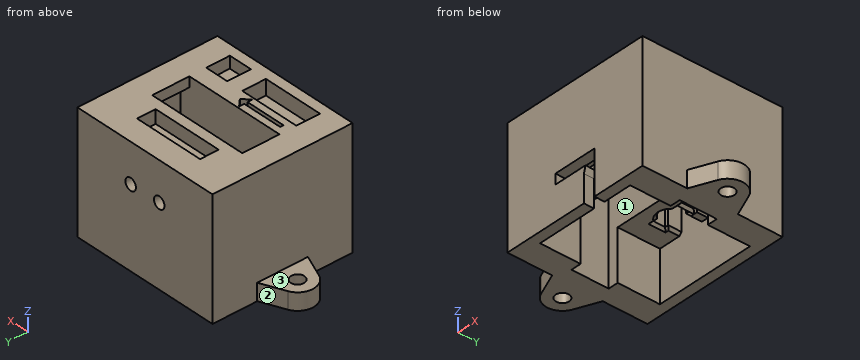
from build123d import *

# Parameters (mm, degrees)
F0_W      = 45
F0_H      = 41.5
F0_W_2    = 18
F0_H_2    = 4
F0_W_3    = 7
F0_H_3    = 3
F0_W_4    = 30
F0_H_4    = 11
F0_W_5    = 8
F0_H_5    = 3.5
F1_DEPTH  = 35
F2_W      = 21
F2_H      = 5.5
F3_DEPTH  = 4
F4_R      = 1.75
F5_DEPTH  = 25
F7_DEPTH  = 4
F9_START  = -8
F8_R      = 3.25
F9_DEPTH  = 17
F11_START = -3
F10_W     = 36
F10_H     = 11
F11_DEPTH = 32.001
F12_W     = 18
F12_H     = 7
F13_DEPTH = 4.5
F14_W     = 7
F14_H     = 4
F15_DEPTH = 3.5
F17_START = -20
F16_W     = 30
F16_H     = 12.5
F16_H_2   = 12
F17_DEPTH = 15.001
F19_DEPTH = 2
F20_R     = 2
F21_DEPTH = 5
F23_DEPTH = 10
F24_SIZE  = 0.74999


# Not quite as in the source:
# - a fillet or chamfer is up to 0.001 mm smaller than in the source, because OpenCascade refuses the exact size


with BuildPart() as f1:
    # F0 (on Top) → F1 (new body)
    with BuildSketch(Plane.XY):
        Rectangle(F0_W, F0_H)
        with Locations((-6, -12.75)):
            Rectangle(F0_W_2, F0_H_2, mode=Mode.SUBTRACT)
        with Locations((11.5, -12.25)):
            Rectangle(F0_W_3, F0_H_3, mode=Mode.SUBTRACT)
        with Locations((0, -0.25)):
            Rectangle(F0_W_4, F0_H_4, mode=Mode.SUBTRACT)
        with Locations((-4.75, 12)):
            Rectangle(F0_W_5, F0_H_5, mode=Mode.SUBTRACT)
        with Locations((4.75, 12)):
            Rectangle(F0_W_5, F0_H_5, mode=Mode.SUBTRACT)
    extrude(amount=F1_DEPTH)

    # F2 (on face) → F3 (cut)
    with BuildSketch(Plane.XY.offset(35)):
        with Locations((0, 11)):
            Rectangle(F2_W, F2_H)
    extrude(amount=-F3_DEPTH, mode=Mode.SUBTRACT)

    # F4 (on face) → F5 (cut)
    with BuildSketch(Plane.XZ.offset(-13.75)):
        with Locations((4.75, 23.5)):
            Circle(F4_R)
        with Locations((-4.75, 23.5)):
            Circle(F4_R)
    extrude(amount=-F5_DEPTH, mode=Mode.SUBTRACT)

    # F6 (on face) → F7 (cut)
    with BuildSketch(Plane.XZ.offset(-13.75)):
        Polygon((4.75, 26.9641016151), (1.75, 25.2320508076), (1.75, 21.7679491924), (1.75, -5.2918036282), (7.75, -5.2918036282), (7.75, 21.7679491924), (7.75, 25.2320508076), align=None)
        Polygon((-1.75, 21.7679491924), (-1.75, 25.2320508076), (-4.75, 26.9641016151), (-7.75, 25.2320508076), (-7.75, 21.7679491924), (-7.75, -5.2918036282), (-1.75, -5.2918036282), align=None)
    extrude(amount=-F7_DEPTH, mode=Mode.SUBTRACT)

    # F8 (on face) → F9 (cut)
    with BuildSketch(Plane.XY.offset(31).offset(F9_START)):
        with Locations((4.75, 12)):
            Circle(F8_R)
        with Locations((-4.75, 12)):
            Circle(F8_R)
    extrude(amount=-F9_DEPTH, mode=Mode.SUBTRACT)

    # F10 (on face) → F11 (cut)
    with BuildSketch(Plane.XY.offset(35).offset(F11_START)):
        with Locations((0, -0.25)):
            Rectangle(F10_W, F10_H)
    extrude(amount=-F11_DEPTH, mode=Mode.SUBTRACT)

    # F12 (on face) → F13 (cut)
    with BuildSketch(Plane.XY.offset(35)):
        with Locations((-6, -14.25)):
            Rectangle(F12_W, F12_H)
    extrude(amount=-F13_DEPTH, mode=Mode.SUBTRACT)

    # F14 (on face) → F15 (cut)
    with BuildSketch(Plane.XY.offset(35)):
        with Locations((11.5, -15.75)):
            Rectangle(F14_W, F14_H)
    extrude(amount=-F15_DEPTH, mode=Mode.SUBTRACT)

    # F16 (on face) → F17 (cut)
    with BuildSketch(Plane.XY.offset(35).offset(F17_START)):
        with Locations((0, 11.5)):
            Rectangle(F16_W, F16_H)
        with Locations((0, -11.75)):
            Rectangle(F16_W, F16_H_2)
    extrude(amount=-F17_DEPTH, mode=Mode.SUBTRACT)

    # F18 (on face) → F19 (cut)
    with BuildSketch(Plane.XY.offset(35)):
        Polygon((-1, -7.75), (-13, -7.75), (-13, -8.75), (-1, -8.75), (-1, -10.25), (1, -8.25), (-1, -6.25), align=None)
    extrude(amount=-F19_DEPTH, mode=Mode.SUBTRACT)

    # F20 (on Top) → F21 (join)
    with BuildSketch(Plane.XY):
        with BuildLine():
            Line((22.5, -7.5), (29.4230769231, -4.6153846154))
            ThreePointArc((29.4230769231, -4.6153846154), (32.5, 0), (29.4230769231, 4.6153846154))
            Line((29.4230769231, 4.6153846154), (22.5, 7.5))
            Line((22.5, 7.5), (22.5, -7.5))
        make_face()
        with Locations((27.5, 0)):
            Circle(F20_R, mode=Mode.SUBTRACT)
        with BuildLine():
            Line((-29.4230769231, -4.6153846154), (-22.5, -7.5))
            Line((-22.5, -7.5), (-22.5, 7.5))
            Line((-22.5, 7.5), (-29.4230769231, 4.6153846154))
            ThreePointArc((-29.4230769231, 4.6153846154), (-32.5, 0), (-29.4230769231, -4.6153846154))
        make_face()
        with Locations((-27.5, 0)):
            Circle(F20_R, mode=Mode.SUBTRACT)
    extrude(amount=F21_DEPTH)

    # F22 (on face) → F23 (cut)
    with BuildSketch(Plane.XZ.offset(20.75)):
        Polygon((3, 8), (3, 0), (6.5, 0), (6.5, 13), (-6.5, 13), (-6.5, 10), (3.5, 10), align=None)
    extrude(amount=-F23_DEPTH, mode=Mode.SUBTRACT)

    # F24 (size 0.75 in the source; OpenCascade refuses exactly that, so slightly less here)
    f24_edges = [f1.edges().sort_by_distance(p)[0] for p in [
        (-7.75, 15.75, 15),
        (-4.75, 8.75, 15),
        (8.119306, 10.25, 15),
        (1.380694, 10.25, 15),
        (-1.380694, 10.25, 15),
        (-8.119306, 10.25, 15),
        (-8.75, 12, 15),
        (-8.25, 13.75, 15),
        (-1.25, 13.75, 15),
        (1.25, 13.75, 15),
        (8.25, 13.75, 15),
        (-1.75, 15.75, 15),
        (1.75, 15.75, 15),
        (4.75, 8.75, 15),
        (8.75, 12, 15),
        (7.75, 15.75, 15),
        (-0.75, 12, 15),
        (0.75, 12, 15),
        (4.75, 10.25, 23),
        (-4.75, 10.25, 23),
    ]]
    chamfer(f24_edges, length=F24_SIZE)


solid = f1.part
Here's how the part is built. I have some questions about the finished solid (model axes, mm). Face numbers are marked on the shaded views. A direction names the side the tool comes from. Give positions to 0.01 mm unless a question says otherwise; leave off trailing zeros. Order: outer loops, then holes, each group sorted by start corner. A loop starts at its lowest first (then second) coordinate and runs counter-clockwise, first axis right, second up. Notation, with made-up numbers: (5.25, 62.5) -> (21.25, 62.5) arc R28 cw to (21.25, 96.5) -> close; hole circle Ø2 at (8, -24). An arc over 180 degrees is marked (long way). One line per item, written item: value. Start each with the question number.
1. Imagine slicing it at A-A, the plane y = 3. List the corners of the cut face in (x, z) for me, plus the area to 3 significant figures.
2. Will these pins go through, and if not, where does the flat tip stop? pin 1 Ø5 at (x, y) = (7.5, 10) entering from +Z; pin 2 Ø8 at (y, z) = (-2, 12) entering from +X; pin 3 Ø3 at (x, y) = (7.5, 8) entering from -Z; pin 4 Ø1.5 at (x, y) = (25.5, 5) entering from +Z.
3. Imagine slicing it at B-B, the plane z = 4. Count the separate pieces of the cut face and the enclosed holes in it, plus the area to 3 significant figures.
4. For the marked faces 1, 2 and 3, which set-ups out of +Z, -Z, +X, -X, +Y, -Y let a thin tool reach every point of the face, with its end or its side?
5. Imagine slicing it at C-C, the plane x = 27.5. List the corners of the cut face in (y, z) for me, plus the area to 3 significant figures.
6. I need wall thicknesses on probe 1 along Y at (x, z) = (-3, 26.5); probe 2 along X at (y, z) = (13.5, 17); probe 3 along Y at (x, z) = (-11, 25.5). Which ranges of each line are inside material? Lowest first, please. Write a range as from..to.
Values follow:
1. outline: (-31.5, 0) -> (-18, 0) -> (-18, 32) -> (-15, 32) -> (-15, 35) -> (-22.5, 35) -> (-22.5, 5) -> (-31.5, 5) -> close; (15, 32) -> (18, 32) -> (18, 0) -> (31.5, 0) -> (31.5, 5) -> (22.5, 5) -> (22.5, 35) -> (15, 35) -> close
1. area: 423 mm2
2. pin 1: stops at z = 35
2. pin 2: stops at x = 22.5
2. pin 3: stops at z = 15
2. pin 4: stops at z = 5
3. separate pieces: 1
3. enclosed holes: 2
3. area: 910 mm2
4. face 1: -Z
4. face 2: +Z, -Z, -X, +Y
4. face 3: +Z, -X, +Y, -Y
5. outline: (-5.42, 0) -> (-2, 0) -> (-2, 5) -> (-5.42, 5) -> close; (2, 0) -> (5.42, 0) -> (5.42, 5) -> (2, 5) -> close
5. area: 34.2 mm2
6. probe 1: y = -20.75..-14.75, -10.75..-5.75, 5.25..10.25, 13.75..20.75
6. probe 2: x = -22.5..-8.75, -0.75..0.75, 8.75..22.5
6. probe 3: y = -20.75..-14.75, -10.75..-5.75, 5.25..20.75
